Autodesk Inventor part; units mm, degrees
ref_plane "YZ Plane" through (0, 0, 0) normal (1, 0, 0) x (0, 1, 0)
ref_plane "XZ Plane" through (0, 0, 0) normal (0, 1, 0) x (-1, 0, 0)
ref_plane "XY Plane" through (0, 0, 0) normal (0, 0, 1) x (1, 0, 0)
sketch "Sketch1" plane through (0, 0, 0) normal (1, 0, 0) x (0, 1, 0)
  line L0 (-40.5, -1.5) -> (40.5, -1.5)
  line L1 (40.5, -1.5) -> (40.5, 1.5)
  line L2 (40.5, 1.5) -> (-40.5, 1.5)
  line L3 (-40.5, 1.5) -> (-40.5, -1.5)
  line L4 (-40.5, -1.5) -> (40.5, 1.5) construction
  line L5 (40.5, -1.5) -> (-40.5, 1.5) construction
  point P0 (0, 0)
  point P1 (0, 0)
  point P2 (0, 0)
  dimension "d27" = 3
  dimension "d28" = 81
extrude "Extrusion1" add sketch "Sketch1" along normal mid plane 88
sketch "Sketch2" plane through (44, 0, 0) normal (1, 0, 0) x (0, 0, -1)
  line L0 (1.5, 40.5) -> (-1.5, 40.5)
  line L1 (-1.5, 40.5) -> (-1.5, -40.5)
  line L2 (-1.5, -40.5) -> (1.5, -40.5)
  line L3 (1.5, -40.5) -> (1.5, 40.5)
  line L4 (1.5, 40.5) -> (-1.5, 40.5)
  line L5 (-1.5, 40.5) -> (-1.5, -127.5)
  line L6 (-1.5, -127.5) -> (1.5, -127.5)
  line L7 (1.5, -127.5) -> (1.5, 40.5)
  line L8 (-1.5, 40.5) -> (-1.5, -40.5)
  point P0 (0, 0)
  dimension "d29" = 168
extrude "Extrusion2" add sketch "Sketch2" along normal blind 40
sketch "Sketch3" plane through (44, -35, 1.5) normal (0, 0, 1) x (1, 0, 0)
  line L0 (-44, 35) -> (111.2969, 35) construction
  line L1 (43, 17.5) -> (40, 17.5)
  line L2 (40, 17.5) -> (40, 52.5)
  line L3 (40, 52.5) -> (43, 52.5)
  line L4 (43, 52.5) -> (43, 17.5)
  line L5 (43, 17.5) -> (40, 52.5) construction
  line L6 (40, 17.5) -> (43, 52.5) construction
  line L7 (40, 75.5) -> (40, -92.5)
  line L8 (0, -5.5) -> (0, -92.5)
  line L9 (0, -92.5) -> (40, -92.5)
  line L10 (40, -92.5) -> (40, 75.5)
  line L11 (40, -8.5) -> (0, -8.5) construction
  line L12 (43, -34.5) -> (40, -34.5)
  line L13 (40, -34.5) -> (40, -69.5)
  line L14 (40, -69.5) -> (43, -69.5)
  line L15 (43, -69.5) -> (43, -34.5)
  line L16 (43, -34.5) -> (40, -69.5) construction
  line L17 (40, -34.5) -> (43, -69.5) construction
  point P0 (41.5, 35)
  point P1 (41.5, -52)
  point P2 (40, -34.5)
  point P3 (40, -69.5)
  dimension "d23" = 3
  dimension "d24" = 35
extrude "Extrusion3" add sketch "Sketch3" against normal up to surface (3 mm away)
mirror "Mirror1" about plane through (0, 0, 0) normal (1, 0, 0) of "Extrusion2", "Extrusion3"
sketch "Sketch4" plane through (84, -127.5, -1.5) normal (0, 0, -1) x (-1, 0, 0)
  line L0 (40, 153) -> (43, 153)
  line L1 (43, 153) -> (43, 138)
  line L2 (43, 138) -> (40, 138)
  line L3 (40, 138) -> (40, 153)
  line L4 (40, 20) -> (43, 20)
  line L5 (43, 55) -> (43, 20)
  line L6 (43, 82.6608) -> (43, 55)
  line L7 (40, 82.6608) -> (43, 82.6608)
  line L8 (40, 55) -> (40, 82.6608)
  line L9 (43, 55) -> (40, 55)
  line L10 (40, 20) -> (40, 55)
  line L11 (40, -14.5469) -> (40, 20)
  line L12 (43, -14.5469) -> (40, -14.5469)
  line L13 (43, 20) -> (43, -14.5469)
  line L14 (125, 153) -> (128, 153)
  line L15 (128, 153) -> (128, 138)
  line L16 (128, 138) -> (125, 138)
  line L17 (125, 138) -> (125, 153)
  line L18 (125, 20) -> (128, 20)
  line L19 (128, 55) -> (128, 20)
  line L20 (128, 82.6608) -> (128, 55)
  line L21 (125, 82.6608) -> (128, 82.6608)
  line L22 (125, 55) -> (125, 82.6608)
  line L23 (128, 55) -> (125, 55)
  line L24 (125, 20) -> (125, 55)
  line L25 (125, -14.5469) -> (125, 20)
  line L26 (128, -14.5469) -> (125, -14.5469)
  line L27 (128, 20) -> (128, -14.5469)
  point P0 (84, 127.5)
extrude "Extrusion4" cut sketch "Sketch4" against normal blind 10 contours L0 L1 L2 L3 | L14 L15 L16 L17
sketch "Sketch5" plane through (44, -127.5, -1.5) normal (0, 0, -1) x (-1, 0, 0)
  line L0 (99.9, 138) -> (99.9, 147)
  line L1 (89.6, 147) -> (89.6, 138)
  line L2 (89.6, 138) -> (99.9, 138)
  line L3 (94.75, 147) -> (94.75, 138) construction
  line L4 (89.75, 147) -> (89.75, 138)
  line L5 (99.75, 138) -> (99.75, 147)
  arc A0 (99.75, 147) -> (89.75, 147) centre (94.75, 147) ccw
  arc A1 (89.75, 138) -> (99.75, 138) centre (94.75, 138) ccw
  point P0 (44, 127.5)
  point P1 (94.75, 142.5)
  dimension "d35" = 10
  dimension "d36" = 9
  dimension "d37" = 0.15
  dimension "d38" = 55.9
  dimension "d39" = 10.5
  dimension "d40" = 9
  dimension "d41" = 9
extrude "Extrusion5" cut sketch "Sketch5" against normal blind 10
sketch "Sketch6" plane through (44, -127.5, 1.5) normal (0, 0, 1) x (1, 0, 0)
  line L0 (-69, 165) -> (-19, 165)
  line L1 (-19, 165) -> (-19, 171)
  line L2 (-19, 171) -> (-69, 171)
  line L3 (-69, 171) -> (-69, 165)
  line L4 (40, 168) -> (-128, 168)
  line L5 (-69, 165) -> (-19, 171) construction
  line L6 (-19, 165) -> (-69, 171) construction
  point P0 (-44, 127.5)
  point P1 (-44, 168)
  point P2 (-69, 168)
  point P3 (-19, 168)
  dimension "d44" = 50
  dimension "d45" = 6
extrude "Extrusion6" add sketch "Sketch6" against normal up to surface (3 mm away) contours L3 L2 L1 L4
properties part number "Suelo"
The listing builds one solid part. Answer for the finished solid, in the listing's coordinates (mm). Coordinates: 2 decimals unless noted, no trailing zeros. Loops run counter-clockwise (first coordinate to the right, second up) from the corner with the lowest first, then second, coordinate; pieces in that order, holes last.
1) Flat-ended cylindrical pins translate along their axes: pin 1 Ø1.5 at (x, z) = (85, 0.5) entering from +Y; pin 2 Ø1 at (y, z) = (-110, 0) entering from -X; pin 3 Ø1.5 at (x, z) = (-56.5, -0.5) entering from +Y. Find the tip coordinate at first contact, or state that the pin passes through.
2) Find section C-C on z = 0.95. Give the number of separate pieces and of enclosed holes in the cut face, then the cut area to 3 significant figures.
3) Find section B-B on y = -59.5. Write down the section's boundary in (x, z), then the cut area to 3 significant figures.
4) Determine the mould class of faces 1 (the face through (-50.64, 5.5, -0.02)), 2 (the face through (-50.86, 24.5, -0.02)), 3 (the face through (-1, -22, 1.5)) for opening direction Y: pulls with the +Y half, pulls with the -Y half, needs draft (parallel to the pull), parting line crosses it, or undercut.
5) Find the intervals of material crossed by L1, parallel to X at y = 18, z = -0.5; L2, parallel to X at y = -65, z = 0.2; L3, parallel to Y at x = -41.5, z = 0.85, in increasing order.
6) Find section A-A on x = -50.75. Write down the section's boundary in (y, z).
7) Find section D-D on x = -68.5. Write down the section's boundary in (y, z).
Values:
1. pin 1: stops at y = 17.5
1. pin 2: stops at x = -84
1. pin 3: stops at y = 40.5
2. separate pieces: 1
2. enclosed holes: 3
2. area: 20,900 mm2
3. outline: (-84, -1.5) - (-44, -1.5) - (-44, 1.5) - (-84, 1.5) - close; (44, -1.5) - (84, -1.5) - (84, 1.5) - (44, 1.5) - close
3. area: 240 mm2
4. face 1: undercut
4. face 2: undercut
4. face 3: needs draft
5. L1: x = -84 to -55.75, -45.75 to -44, -41 to 41, 44 to 84
5. L2: x = -84 to -44, 44 to 84
5. L3: y = -40.5 to 10.5, 25.5 to 40.5
6. outline: (-127.5, -1.5) - (5.5, -1.5) - (5.5, 1.5) - (-127.5, 1.5) - close; (24.5, -1.5) - (40.5, -1.5) - (40.5, 1.5) - (24.5, 1.5) - close
7. outline: (-127.5, -1.5) - (40.5, -1.5) - (40.5, 1.5) - (-127.5, 1.5) - close
